Autodesk Inventor part; units mm, degrees
ref_plane "C1_XY" through (0, 0, 0) normal (0, 0, 1) x (1, 0, 0)
ref_plane "C1_YZ" through (0, 0, 0) normal (1, 0, 0) x (0, 1, 0)
ref_plane "C1_ZX" through (0, 0, 0) normal (0, 1, 0) x (0, 0, 1)
sketch "Sketch_75" plane through (0, 0, 0) normal (0, 0, 1) x (1, 0, 0)
  line L0 (-10, -3) -> (-10, -9)
  arc A0 (-10, -9) -> (-9, -10) centre (-9, -9) ccw
  line L1 (-9, -10) -> (-3, -10)
  line L2 (-3, -10) -> (-3, -8)
  line L3 (-3, -8) -> (-6, -8)
  line L4 (-6, -8) -> (-6, -7.0607)
  line L5 (-6, -7.0607) -> (-2.9393, -4)
  line L6 (-2.9393, -4) -> (-0.6536, -4)
  arc A1 (-0.6536, -4) -> (-0.4036, -3.933) centre (-0.6536, -3.5) ccw
  line L7 (-0.4036, -3.933) -> (0, -3.7)
  line L8 (0, -3.7) -> (0.4036, -3.933)
  arc A2 (0.4036, -3.933) -> (0.9036, -3.933) centre (0.6536, -3.5) ccw
  line L9 (0.9036, -3.933) -> (1.2189, -3.751)
  line L10 (1.2189, -3.751) -> (2.5, -4)
  line L11 (2.5, -4) -> (2.9393, -4)
  line L12 (2.9393, -4) -> (6, -7.0607)
  line L13 (6, -7.0607) -> (6, -8)
  line L14 (6, -8) -> (3, -8)
  line L15 (3, -8) -> (3, -10)
  line L16 (3, -10) -> (9, -10)
  arc A3 (9, -10) -> (10, -9) centre (9, -9) ccw
  line L17 (10, -9) -> (10, -3)
  line L18 (10, -3) -> (8, -3)
  line L19 (8, -3) -> (8, -6)
  line L20 (8, -6) -> (7.0607, -6)
  line L21 (7.0607, -6) -> (4, -2.9393)
  line L22 (4, -2.9393) -> (4, -0.6536)
  arc A4 (4, -0.6536) -> (3.933, -0.4036) centre (3.5, -0.6536) ccw
  line L23 (3.933, -0.4036) -> (3.7, 0)
  line L24 (3.7, 0) -> (3.933, 0.4036)
  arc A5 (3.933, 0.4036) -> (3.933, 0.9036) centre (3.5, 0.6536) ccw
  line L25 (3.933, 0.9036) -> (3.751, 1.2189)
  line L26 (3.751, 1.2189) -> (4, 2.5)
  line L27 (4, 2.5) -> (4, 2.9393)
  line L28 (4, 2.9393) -> (7.0607, 6)
  line L29 (7.0607, 6) -> (8, 6)
  line L30 (8, 6) -> (8, 3)
  line L31 (8, 3) -> (10, 3)
  line L32 (10, 3) -> (10, 9)
  arc A6 (10, 9) -> (9, 10) centre (9, 9) ccw
  line L33 (9, 10) -> (3, 10)
  line L34 (3, 10) -> (3, 8)
  line L35 (3, 8) -> (6, 8)
  line L36 (6, 8) -> (6, 7.0607)
  line L37 (6, 7.0607) -> (2.9393, 4)
  line L38 (2.9393, 4) -> (0.6536, 4)
  arc A7 (0.6536, 4) -> (0.4036, 3.933) centre (0.6536, 3.5) ccw
  line L39 (0.4036, 3.933) -> (0, 3.7)
  line L40 (0, 3.7) -> (-0.4036, 3.933)
  arc A8 (-0.4036, 3.933) -> (-0.9036, 3.933) centre (-0.6536, 3.5) ccw
  line L41 (-0.9036, 3.933) -> (-1.2189, 3.751)
  line L42 (-1.2189, 3.751) -> (-2.5, 4)
  line L43 (-2.5, 4) -> (-2.9393, 4)
  line L44 (-2.9393, 4) -> (-6, 7.0607)
  line L45 (-6, 7.0607) -> (-6, 8)
  line L46 (-6, 8) -> (-3, 8)
  line L47 (-3, 8) -> (-3, 10)
  line L48 (-3, 10) -> (-9, 10)
  arc A9 (-9, 10) -> (-10, 9) centre (-9, 9) ccw
  line L49 (-10, 9) -> (-10, 3)
  line L50 (-10, 3) -> (-8, 3)
  line L51 (-8, 3) -> (-8, 6)
  line L52 (-8, 6) -> (-7.0607, 6)
  line L53 (-7.0607, 6) -> (-4, 2.9393)
  line L54 (-4, 2.9393) -> (-4, 0.6536)
  arc A10 (-4, 0.6536) -> (-3.933, 0.4036) centre (-3.5, 0.6536) ccw
  line L55 (-3.933, 0.4036) -> (-3.7, 0)
  line L56 (-3.7, 0) -> (-3.933, -0.4036)
  arc A11 (-3.933, -0.4036) -> (-3.933, -0.9036) centre (-3.5, -0.6536) ccw
  line L57 (-3.933, -0.9036) -> (-3.751, -1.2189)
  line L58 (-3.751, -1.2189) -> (-4, -2.5)
  line L59 (-4, -2.5) -> (-4, -2.9393)
  line L60 (-4, -2.9393) -> (-7.0607, -6)
  line L61 (-7.0607, -6) -> (-8, -6)
  line L62 (-8, -6) -> (-8, -3)
  line L63 (-8, -3) -> (-10, -3)
extrude "Extrusion1" add sketch "Sketch_75" against normal blind 120
sketch "Sketch2" plane through (0, 0, -120) normal (0, 0, -1) x (-1, 0, 0)
  point P0 (0, 0)
hole "Hole1" at (0, 0, -120) direction (0, 0, 1) diameter 4.2 depth 100
ref_plane "C1_XY" through (0, 0, 0) normal (0, 0, 1) x (1, 0, 0)
ref_plane "C1_YZ" through (0, 0, 0) normal (1, 0, 0) x (0, 1, 0)
ref_plane "C1_ZX" through (0, 0, 0) normal (0, 1, 0) x (0, 0, 1)
properties part number "NFS5-2020-100" material "アルミニウム 6061"
Design review of the part built by this model. Coordinates are the model's own, in mm. A direction names the side the tool comes from. Give positions to 0.01 mm unless a question says otherwise; leave off trailing zeros. Write each loop counter-clockwise with the first axis right and the second up, starting at its lowest first coordinate (ties: lowest second). Pieces come first, ordered by that corner, then holes. Notation, with made-up numbers: (59, -20) -> (95, -20) arc R26 ccw to (95, 12) -> close; hole circle Ø5 at (32, 71). An arc over 180 degrees is marked (long way). Answer in a Markdown table with one row per item.
(1) To check wall thickness, follow probe 1 along Y at (x, z) = (0, -91.5); probe 2 along Y at (x, z) = (7.75, -40). State the ranges of each line that lie inside material, in increasing order.
Results:
| item | result |
|---|---|
| probe 1 | -3.7 to -2.1, 2.1 to 3.7 |
| probe 2 | -10 to -6, 6 to 10 |
(2) Clearance check with flat-ended pins moving along their axes: pin 1 (2 mm diameter, centred on y = -1.5, z = -15.5, fed in from -X); pin 2 (0.5 mm diameter, centred on x = 2.5, z = -38, fed in from -Y); pin 3 (0.7 mm diameter, centred on y = -1.5, z = -43, fed in from +X). State where each tip first meets the part, or that it passes through.
Results:
| item | result |
|---|---|
| pin 1 | x = -4 |
| pin 2 | y = -4 |
| pin 3 | x = 4 |
(3) For faces 1 (the flat face through (9, -3, -59)), 2 (the flat face through (4, 8, -59)), 3 (the flat face through (2, 4, -59)), 4 (the cylindrical face through (-0.631, 2.003, -69.3)), 5 (the flat face through (-2, -4, -59)), list the 3-axis set-ups (+Z, -Z, +X, -X, +Y, -Y) from which the entire face can be reached by the end or side of a thin tool; tool diameter is ignored.
Results:
| item | result |
|---|---|
| face 1 | +Z, -Z, +X |
| face 2 | +Z, -Z |
| face 3 | +Z, -Z, +Y |
| face 4 | -Z |
| face 5 | +Z, -Z, -Y |
(4) Mouldability with a two-part tool opening along X and no side actions: class faces 6 (the flat face through (-0.1, 2.4, -120)), 7 (the flat face through (10, 6, -59)), 8 (the flat face through (-4, -8, -59)) as +X half, -X half, draft (parallel to the pull), parting line (faces both ways), or undercut.
Results:
| item | result |
|---|---|
| face 6 | draft |
| face 7 | +X half |
| face 8 | undercut |
(5) Consider section A-A (y = -5). State the section outline as (x, z) points, then the cut area to 3 significant figures.
Results:
| item | result |
|---|---|
| outline | (-10, -120) -> (-8, -120) -> (-8, 0) -> (-10, 0) -> close; (-6.06, -120) -> (-3.94, -120) -> (-3.94, 0) -> (-6.06, 0) -> close; (3.94, -120) -> (6.06, -120) -> (6.06, 0) -> (3.94, 0) -> close; (8, -120) -> (10, -120) -> (10, 0) -> (8, 0) -> close |
| area | 989 mm2 |
